The model under review builds one solid part; all positions refer to its coordinate system, in mm. A direction names the side the tool comes from. Round coordinates to 2 decimals unless told otherwise and drop trailing zeros. Loops run counter-clockwise (first coordinate to the right, second up) from the corner with the lowest first, then second, coordinate; pieces in that order, holes last. Notation, with made-up numbers: M 47,-33 L 88,-33 A17 ccw 88,-24 Z; hole C -26,26.25 d1. An arc over 180 degrees is marked long. Answer as a JSON object with one key per item and string values. Group by question number.
Item 1: To check wall thickness, follow line 1 (Z direction, x = 25, y = -28); line 2 (Y direction, x = -40, z = 117). State the ranges of each line that lie inside material, in increasing order.
Item 2: Insertion check: P1, Ø1.7, axis at x = 1, y = -41, coming from the -Z side; P2, Ø3, axis at x = 3, z = 149, coming from the +Y side; P3, Ø10, axis at x = -22, y = -22.5, coming from the +Z side. Each pin has a flat end and moves straight along its axis. Give the tip position at first contact, or say it passes through.
Item 3: The part is to be moulded in two halves that separate along X. For faces 3 (the face through (-42.36, 2.16, 152.9)), 4 (the face through (-0.417, -36.827, 152.9)), 5 (the face through (40, 0, 305)), say which applies: +X half, -X half, draft (parallel to the pull), parting line (faces both ways), or undercut.
Item 4: Consider section D-D (x = -24). Give the boundary of the cut face in (y, z), and give its area (3 significant figures).
Item 5: Consider section C-C (z = 157). Give the boundary of the cut face in (x, y).
Item 6: Tool access review of faces 1 (the face through (-0.417, 43.173, 152.9)), 2 (the face through (0, -40, 305)): name each direction out of +Z, -Z, +X, -X, +Y, -Y from which nothing blocks a thin tool from reaching the whole face with its end or side.
Item 7: Consider section A-A (y = 0). Give the boundary of the cut face in (x, z), and give its area (3 significant figures).
```python
from build123d import *

# Parameters (mm, degrees)
F0_R     = 40
F1_DEPTH = 5
F2_R     = 3.2
F3_DEPTH = 300


with BuildPart() as f1:
    # F0 (on Top) → F1 (new body)
    with BuildSketch(Plane.XY):
        Circle(F0_R)
    extrude(amount=F1_DEPTH)

    # F2 (on face) → F3 (join)
    with BuildSketch(Plane.XY.offset(5)):
        with Locations((0, 40)):
            Circle(F2_R)
        with Locations((-40, 0)):
            Circle(F2_R)
        with Locations((0, -40)):
            Circle(F2_R)
        with Locations((40, 0)):
            Circle(F2_R)
    extrude(amount=F3_DEPTH)


solid = f1.part
```
Geometry results:
{
 "1": {"line 1": "z = 0 to 5", "line 2": "y = -3.2 to 3.2"},
 "2": {"P1": "stops at z = 5", "P2": "stops at y = 42.83", "P3": "stops at z = 5"},
 "3": {"face 3": "undercut", "face 4": "parting line", "face 5": "draft"},
 "4": {"outline": "M -32,0 L 32,0 L 32,5 L -32,5 Z", "area": "320 mm^2"},
 "5": {"outline": "C -40,0 d6.4; C 0,-40 d6.4; C 0,40 d6.4; C 40,0 d6.4"},
 "6": {"face 1": "+Z", "face 2": "+Z, +X, -X, +Y, -Y"},
 "7": {"outline": "M -43.2,5 L -40,5 L -40,0 L 40,0 L 40,5 L 43.2,5 L 43.2,305 L 36.8,305 L 36.8,5 L -36.8,5 L -36.8,305 L -43.2,305 Z", "area": "4,240 mm^2"}
}
